Source: CAD feature listing. Evaluate the final solid. Frame: model axes, mm. A direction names the side the tool comes from. Coordinates: 2 decimals unless noted, no trailing zeros. Order: outer loops, then holes, each group sorted by start corner. A loop starts at its lowest first (then second) coordinate and runs counter-clockwise, first axis right, second up.
```python
from build123d import *

# Parameters (mm, degrees)
SKETCH1_R           = 20
BOSS_EXTRUDE1_DEPTH = 70
CUT_EXTRUDE1_DEPTH  = 71
CIRPATTERN1_COUNT   = 22
SKETCH3_R           = 23
BOSS_EXTRUDE2_DEPTH = 10
SKETCH5_R           = 23
BOSS_EXTRUDE3_DEPTH = 10
SKETCH6_R           = 7.5
CUT_EXTRUDE2_DEPTH  = 81
FILLET1_R           = 2


with BuildPart() as part:
    # Sketch1 → Boss-Extrude1 (new body)
    with BuildSketch(Plane.XY):
        Circle(SKETCH1_R)
    extrude(amount=BOSS_EXTRUDE1_DEPTH)

    # Sketch2 → Cut-Extrude1 (cut, through all)
    with BuildSketch(Plane.XY.offset(70)):
        with BuildLine():
            Line((-1.3875, 18.447895375), (1.3875, 18.447895375))
            Line((1.3875, 18.447895375), (1.5, 19.943670675))
            ThreePointArc((1.5, 19.943670675), (0, 20), (-1.5, 19.943670675))
            Line((-1.5, 19.943670675), (-1.3875, 18.447895375))
        make_face()
    cut_extrude1 = extrude(amount=-CUT_EXTRUDE1_DEPTH, mode=Mode.SUBTRACT)

    # CirPattern1: Cut-Extrude1 ×22 about axis
    cirpattern1_axis = Axis((0, 0, 0), (0, 0, 1))
    for i in range(1, CIRPATTERN1_COUNT):
        add(cut_extrude1.rotate(cirpattern1_axis, i * 360 / CIRPATTERN1_COUNT), mode=Mode.SUBTRACT)

    # Sketch3 → Boss-Extrude2 (add)
    with BuildSketch(Plane.XY.offset(70)):
        Circle(SKETCH3_R)
    extrude(amount=-BOSS_EXTRUDE2_DEPTH)

    # Sketch5 → Boss-Extrude3 (add)
    with BuildSketch(Plane(origin=(0, 0, 0), x_dir=(-1, 0, 0), z_dir=(0, 0, -1))):
        Circle(SKETCH5_R)
    extrude(amount=BOSS_EXTRUDE3_DEPTH)

    # Sketch6 → Cut-Extrude2 (cut, through all)
    with BuildSketch(Plane.XY.offset(70)):
        Circle(SKETCH6_R)
    extrude(amount=-CUT_EXTRUDE2_DEPTH, mode=Mode.SUBTRACT)

    # Fillet1
    fillet1_edges = [part.edges().sort_by_distance(p)[0] for p in [
        (-23, 0, 70),
        (-23, 0, 60),
        (23, 0, 0),
        (23, 0, -10),
    ]]
    fillet(fillet1_edges, radius=FILLET1_R)


solid = part.part
```
Q1. Pin query (flat end, axial travel): P1, Ø12, axis at x = 0, y = 0, coming from the -Z side; P2, Ø2, axis at x = -2, z = 28.5, coming from the -Y side; P3, Ø3, axis at y = -8.5, z = 25.5, coming from the -X side; P4, Ø2, axis at x = -13.5, z = 30, coming from the -Y side. Return the tip coordinate at first contact, or that it passes through.
Solutions:
P1: passes through
P2: stops at y = -19.94
P3: stops at x = -17.52
P4: stops at y = -15.61
Q2. Section query C-C on z = -3. Output: boundary loops of the cut face in (x, y).
Solutions:
outline: circle Ø46 at (0, 0); hole circle Ø15 at (0, 0)
Q3. Set-up query: faces 1 (the cylindrical face through (-19.2, -5.6, 29.6)), 2 (the cylindrical face through (13.112, 15.103, 29.58)), 3 (the cylindrical face through (8.29, -18.2, 29.58)), 4 (the cylindrical face through (-16.815, 10.829, 29.58)), 5 (the flat face through (-16.773, -7.681, 30.42)). Return all of +Z, -Z, +X, -X, +Y, -Y with unobstructed straight access to the full face (end or side cutting, diameter ignored); none if empty.
Solutions:
face 1: -X, -Y
face 2: +X, +Y
face 3: +X, -Y
face 4: -X, +Y
face 5: none
Q4. Section query A-A on x = 0. Output: boundary loops of the cut face in (y, z), plus the area to 3 significant figures.
Solutions:
outline: (-23, -8) arc R2 ccw to (-21, -10) - (-7.5, -10) - (-7.5, 70) - (-21, 70) arc R2 ccw to (-23, 68) - (-23, 62) arc R2 ccw to (-21, 60) - (-18.45, 60) - (-18.45, 0) - (-21, 0) arc R2 ccw to (-23, -2) - close; (7.5, -10) - (21, -10) arc R2 ccw to (23, -8) - (23, -2) arc R2 ccw to (21, 0) - (18.45, 0) - (18.45, 60) - (21, 60) arc R2 ccw to (23, 62) - (23, 68) arc R2 ccw to (21, 70) - (7.5, 70) - close
area: 1,930 mm2
Q5. Pull-direction query (X, two-part tool) for faces 6 (the cylindrical face through (-8.326, -18.185, 29.58)), 7 (the flat face through (13.929, 12.095, 30.42)), 8 (the cylindrical face through (2.83, -19.8, 29.58)); classes: pulls with the +X half, pulls with the -X half, needs draft (parallel to the pull), parting line crosses it, or undercut.
Solutions:
face 6: pulls with the -X half
face 7: undercut
face 8: pulls with the +X half
Q6. Section query B-B on y = 0. Output: boundary loops of the cut face in (x, z), plus the area to 3 significant figures.
Solutions:
outline: (-23, -8) arc R2 ccw to (-21, -10) - (-7.5, -10) - (-7.5, 70) - (-21, 70) arc R2 ccw to (-23, 68) - (-23, 62) arc R2 ccw to (-21, 60) - (-20, 60) - (-20, 0) - (-21, 0) arc R2 ccw to (-23, -2) - close; (7.5, -10) - (21, -10) arc R2 ccw to (23, -8) - (23, -2) arc R2 ccw to (21, 0) - (20, 0) - (20, 60) - (21, 60) arc R2 ccw to (23, 62) - (23, 68) arc R2 ccw to (21, 70) - (7.5, 70) - close
area: 2,110 mm2
Q7. Material intervals for line 1 along Y through (x, z) = (0, 16.5); line 2 along X through (y, z) = (-11.5, 55); line 3 along Z through (x, y) = (19, -6.5), sorted ascending.
Solutions:
line 1: y = -18.45 to -7.5, 7.5 to 18.45
line 2: x = -16.36 to -15.48, -14.45 to 14.45, 15.48 to 16.36
line 3: z = -10 to 0, 60 to 70
